Autodesk Inventor part; units mm, degrees
ref_plane "YZ Plane" through (0, 0, 0) normal (1, 0, 0) x (0, 1, 0)
ref_plane "XZ Plane" through (0, 0, 0) normal (0, 1, 0) x (-1, 0, 0)
ref_plane "XY Plane" through (0, 0, 0) normal (0, 0, 1) x (1, 0, 0)
sketch "Sketch1" plane through (0, 0, 0) normal (0, 0, 1) x (1, 0, 0)
  line L0 (3.7674, 2.461) -> (4.3315, 3.068) construction
  line L1 (4.3315, 3.068) -> (2.5, 4.7697) construction
  line L2 (2.5, 4.7697) -> (2.94, 6) construction
  line L3 (2.94, 6) -> (-2, 6) construction
  line L4 (-2, 6) -> (-2, 4.0311) construction
  arc A0 (-2, 4.0311) -> (-3.182, 3.182) centre (0, 0) ccw construction
  line L5 (-3.182, 3.182) -> (-3.182, -3.182) construction
  line L6 (-3.182, -3.182) -> (3.182, -3.182) construction
  arc A1 (3.182, -3.182) -> (3.7674, 2.461) centre (0, 0) ccw construction
  circle A2 centre (0, 0) radius 1.2484
  circle A3 centre (0, 3) radius 0.7934
  circle A4 centre (1.875, -1.75) radius 0.7934
  circle A5 centre (-1.875, -1.75) radius 0.7934
  circle A6 centre (0, 0) radius 4 construction
  line L7 (-2, -4.0311) -> (-2, -3.182) construction
  arc A7 (-2, -4.0311) -> (3.182, -3.182) centre (0, 0) ccw construction
  line L8 (-2, -3.182) -> (3.182, -3.182) construction
  arc A8 (-2, 4.0311) -> (-2, -4.0311) centre (0, 0) ccw construction
  line L9 (-3.182, 3.182) -> (-4.182, 3.182) construction
  line L10 (-4.182, 3.182) -> (-4.182, 4.182) construction
  line L11 (-4.182, 4.182) -> (-3.182, 4.182) construction
  line L12 (-3.182, 4.182) -> (-3.182, 3.182) construction
  line L13 (3.182, -3.182) -> (4.182, -3.182) construction
  line L14 (4.182, -3.182) -> (4.182, -4.182) construction
  line L15 (4.182, -4.182) -> (3.182, -4.182) construction
  line L16 (3.182, -4.182) -> (3.182, -3.182) construction
  line L17 (4.182, -4.182) -> (-4.182, -4.182) construction
  line L18 (-4.182, -4.182) -> (-4.182, -3.182) construction
  line L19 (-4.182, -3.182) -> (4.182, -3.182) construction
  line L20 (4.182, -3.182) -> (4.182, -4.182) construction
  line L21 (-4.182, 4.182) -> (-3.182, 4.182) construction
  line L22 (-3.182, 4.182) -> (-3.182, -4.182) construction
  line L23 (-3.182, -4.182) -> (-4.182, -4.182) construction
  line L24 (-4.182, -4.182) -> (-4.182, 4.182) construction
  line L25 (4.3315, 3.068) -> (6.7138, 5.632) construction
  line L26 (4.3315, 3.068) -> (4.6718, 3.4343) construction
  line L27 (4.6718, 3.4343) -> (2.6832, 5.282) construction
  line L28 (6.7138, 5.632) -> (4.8824, 7.3337) construction
  line L29 (2.5, 4.7697) -> (4.8824, 7.3337) construction
  line L30 (2.8403, 5.136) -> (-3.182, 4.182) construction
  line L31 (4.6718, 3.4343) -> (4.182, -3.182) construction
  circle A9 centre (-3.182, -3.182) radius 0.5 construction
  line L32 (-4.182, 4.182) -> (-4.182, -4.182)
  line L33 (-4.182, -4.182) -> (4.182, -4.182)
  line L34 (4.182, -4.182) -> (4.6718, 3.4343)
  line L35 (6.7138, 5.632) -> (4.6718, 3.4343)
  line L36 (6.7138, 5.632) -> (4.9203, 7.2985)
  line L37 (4.9203, 7.2985) -> (2.8403, 5.136)
  line L38 (2.8403, 5.136) -> (-4.182, 4.182)
  dimension "d0" = 1
  dimension "d1" = 1
  dimension "d2" = 1
  dimension "d3" = 1
  dimension "d4" = 3.5
  dimension "d5" = 0.5
extrude "Extrusion1" add sketch "Sketch1" along normal blind 1
sketch "Sketch2" plane through (0, 0, 1) normal (0, 0, 1) x (1, 0, 0)
  circle A0 centre (0, 0) radius 1.2484
  circle A1 centre (0, 3) radius 0.7934
  line L0 (-3.182, -3.182) -> (3.182, -3.182) construction
  circle A2 centre (0, 0) radius 4 construction
  line L1 (-3.182, 3.182) -> (-3.182, -3.182) construction
  arc A3 (-2, 4.0311) -> (-2, -4.0311) centre (0, 0) ccw construction
  arc A4 (-2, 4.0311) -> (-3.182, 3.182) centre (0, 0) ccw construction
  arc A5 (3.182, -3.182) -> (3.7674, 2.461) centre (0, 0) ccw construction
  line L2 (3.7674, 2.461) -> (4.3315, 3.068) construction
  line L3 (4.3315, 3.068) -> (2.5, 4.7697) construction
  line L4 (-2, -3.182) -> (3.182, -3.182) construction
  arc A6 (-2, -4.0311) -> (3.182, -3.182) centre (0, 0) ccw construction
  line L5 (-2, -4.0311) -> (-2, -3.182) construction
  circle A7 centre (-1.875, -1.75) radius 0.7934
  line L6 (-2, 6) -> (-2, 4.0311) construction
  line L7 (2.5, 4.7697) -> (2.94, 6) construction
  line L8 (2.94, 6) -> (-2, 6) construction
  circle A8 centre (1.875, -1.75) radius 0.7934
  line L9 (-3.182, 3.182) -> (-4.182, 3.182) construction
  line L10 (-4.182, 3.182) -> (-4.182, 4.182) construction
  line L11 (-4.182, 4.182) -> (-3.182, 4.182) construction
  line L12 (-3.182, 4.182) -> (-3.182, 3.182) construction
  line L13 (3.182, -3.182) -> (4.182, -3.182) construction
  line L14 (4.182, -3.182) -> (4.182, -4.182) construction
  line L15 (4.182, -4.182) -> (3.182, -4.182) construction
  line L16 (3.182, -4.182) -> (3.182, -3.182) construction
  line L17 (4.182, -4.182) -> (-4.182, -4.182) construction
  line L18 (-4.182, -4.182) -> (-4.182, -3.182) construction
  line L19 (-4.182, -3.182) -> (4.182, -3.182) construction
  line L20 (4.182, -3.182) -> (4.182, -4.182) construction
  line L21 (-4.182, 4.182) -> (-3.182, 4.182) construction
  line L22 (-3.182, 4.182) -> (-3.182, -4.182) construction
  line L23 (-3.182, -4.182) -> (-4.182, -4.182) construction
  line L24 (-4.182, -4.182) -> (-4.182, 4.182) construction
  line L25 (4.3315, 3.068) -> (6.7138, 5.632) construction
  line L26 (4.3315, 3.068) -> (4.6718, 3.4343) construction
  line L27 (4.6718, 3.4343) -> (2.6832, 5.282) construction
  line L28 (6.7138, 5.632) -> (4.8824, 7.3337) construction
  line L29 (2.5, 4.7697) -> (4.8824, 7.3337) construction
  line L30 (2.8403, 5.136) -> (-3.182, 4.182) construction
  line L31 (4.6718, 3.4343) -> (4.182, -3.182) construction
  arc A9 (-3.182, -2.682) -> (-2.682, -3.182) centre (-3.182, -3.182) ccw
  line L32 (-4.182, 4.182) -> (-4.182, -4.182)
  line L33 (-4.182, -4.182) -> (4.182, -4.182)
  line L34 (4.182, -4.182) -> (4.6718, 3.4343)
  line L35 (6.7138, 5.632) -> (4.6718, 3.4343)
  line L36 (6.7138, 5.632) -> (4.9203, 7.2985)
  line L37 (4.9203, 7.2985) -> (2.8403, 5.136)
  line L38 (2.8403, 5.136) -> (-4.182, 4.182)
  line L39 (-3.182, -2.682) -> (-3.182, 4.3178)
  line L40 (2.8403, 5.136) -> (-4.182, 4.182)
  line L41 (-2.682, -3.182) -> (4.2463, -3.182)
  dimension "d8" = 1
  dimension "d9" = 1
  dimension "d10" = 1
  dimension "d11" = 1
  dimension "d12" = 3.5
  dimension "d13" = 0.5
extrude "Extrusion2" add sketch "Sketch2" along normal blind 2.5 contours A9 L41 L34 L33 L32 L38 L39
sketch "Sketch3" plane through (0, 0, 1) normal (0, 0, 1) x (1, 0, 0)
  circle A0 centre (0, 0) radius 1.2484
  circle A1 centre (0, 3) radius 0.7934
  line L0 (-3.182, -3.182) -> (3.182, -3.182) construction
  circle A2 centre (0, 0) radius 4 construction
  line L1 (-3.182, 3.182) -> (-3.182, -3.182) construction
  arc A3 (-2, 4.0311) -> (-2, -4.0311) centre (0, 0) ccw construction
  arc A4 (-2, 4.0311) -> (-3.182, 3.182) centre (0, 0) ccw construction
  arc A5 (3.182, -3.182) -> (3.7674, 2.461) centre (0, 0) ccw construction
  line L2 (3.7674, 2.461) -> (4.3315, 3.068) construction
  line L3 (4.3315, 3.068) -> (2.5, 4.7697) construction
  line L4 (-2, -3.182) -> (3.182, -3.182) construction
  arc A6 (-2, -4.0311) -> (3.182, -3.182) centre (0, 0) ccw construction
  line L5 (-2, -4.0311) -> (-2, -3.182) construction
  circle A7 centre (-1.875, -1.75) radius 0.7934
  line L6 (-2, 6) -> (-2, 4.0311) construction
  line L7 (2.5, 4.7697) -> (2.94, 6) construction
  line L8 (2.94, 6) -> (-2, 6) construction
  circle A8 centre (1.875, -1.75) radius 0.7934
  line L9 (-3.182, 3.182) -> (-4.182, 3.182) construction
  line L10 (-4.182, 3.182) -> (-4.182, 4.182) construction
  line L11 (-4.182, 4.182) -> (-3.182, 4.182) construction
  line L12 (-3.182, 4.182) -> (-3.182, 3.182) construction
  line L13 (3.182, -3.182) -> (4.182, -3.182) construction
  line L14 (4.182, -3.182) -> (4.182, -4.182) construction
  line L15 (4.182, -4.182) -> (3.182, -4.182) construction
  line L16 (3.182, -4.182) -> (3.182, -3.182) construction
  line L17 (4.182, -4.182) -> (-4.182, -4.182) construction
  line L18 (-4.182, -4.182) -> (-4.182, -3.182) construction
  line L19 (-4.182, -3.182) -> (4.182, -3.182) construction
  line L20 (4.182, -3.182) -> (4.182, -4.182) construction
  line L21 (-4.182, 4.182) -> (-3.182, 4.182) construction
  line L22 (-3.182, 4.182) -> (-3.182, -4.182) construction
  line L23 (-3.182, -4.182) -> (-4.182, -4.182) construction
  line L24 (-4.182, -4.182) -> (-4.182, 4.182) construction
  line L25 (4.3315, 3.068) -> (6.7138, 5.632) construction
  line L26 (4.3315, 3.068) -> (4.6718, 3.4343) construction
  line L27 (4.6718, 3.4343) -> (2.6832, 5.282) construction
  line L28 (6.7138, 5.632) -> (4.8824, 7.3337) construction
  line L29 (2.5, 4.7697) -> (4.8824, 7.3337) construction
  line L30 (2.8403, 5.136) -> (-3.182, 4.182) construction
  line L31 (4.6718, 3.4343) -> (4.182, -3.182) construction
  circle A9 centre (-3.182, -3.182) radius 0.5 construction
  line L32 (-4.182, 4.182) -> (-4.182, -4.182)
  line L33 (-4.182, -4.182) -> (4.182, -4.182)
  line L34 (4.182, -4.182) -> (4.6718, 3.4343)
  line L35 (6.7138, 5.632) -> (4.6718, 3.4343)
  line L36 (6.7138, 5.632) -> (4.9203, 7.2985)
  line L37 (4.9203, 7.2985) -> (2.8403, 5.136)
  line L38 (2.8403, 5.136) -> (-4.182, 4.182)
  line L39 (2.8403, 5.136) -> (-3.182, 4.3178)
  line L40 (4.2463, -3.182) -> (4.6718, 3.4343)
  line L41 (2.8403, 5.136) -> (4.6718, 3.4343)
  dimension "d16" = 1
  dimension "d17" = 1
  dimension "d18" = 1
  dimension "d19" = 1
  dimension "d20" = 3.5
  dimension "d21" = 0.5
extrude "Extrusion3" add sketch "Sketch3" along normal blind 2 contours L37 L36 L35 L41
sketch "Sketch4" plane through (4.9203, 7.2985, 3) normal (0.6807, 0.7326, 0) x (0.7326, -0.6807, 0)
  line L0 (2.4482, 2) -> (-0.0518, 2) construction
  line L1 (2.4482, 2) -> (2.4482, 0) construction
  line L2 (-0.0518, 0) -> (2.4482, 0) construction
  line L3 (-0.0518, 2) -> (-0.0518, 0) construction
  line L4 (2.4482, 0) -> (0, 0) construction
  line L5 (1.2241, 0) -> (-0.0518, 0) construction
  line L6 (-0.0518, 0) -> (-0.0518, 1) construction
  line L7 (-0.0518, 1) -> (1.2241, 1) construction
  line L8 (1.2241, 1) -> (1.2241, 0) construction
  circle A0 centre (1.2241, 1) radius 0.65
  dimension "d24" = 1.3
extrude "Extrusion4" cut sketch "Sketch4" against normal blind 3
sketch "Sketch5" plane through (0, 0, 0) normal (0, 0, -1) x (-1, 0, 0)
  line L0 (4.182, 4.182) -> (4.182, -4.182)
  line L1 (4.182, -4.182) -> (-4.182, -4.182)
  line L2 (-4.182, -4.182) -> (-4.2463, -3.182)
  line L3 (-4.2463, -3.182) -> (2.682, -3.182)
  arc A0 (2.682, -3.182) -> (3.182, -2.682) centre (3.182, -3.182) ccw
  line L4 (3.182, -2.682) -> (3.182, 4.3178)
  line L5 (3.182, 4.3178) -> (4.182, 4.182)
  point P0 (0, 0)
extrude "Extrusion5" add sketch "Sketch5" along normal blind 2.5
sketch "Sketch6" plane through (0, 0, 0) normal (0, 0, -1) x (-1, 0, 0)
  line L0 (-6.7138, 5.632) -> (-4.9203, 7.2985)
  line L1 (-4.9203, 7.2985) -> (-2.8403, 5.136)
  line L2 (-2.8403, 5.136) -> (-4.6718, 3.4343)
  line L3 (-4.6718, 3.4343) -> (-6.7138, 5.632)
  point P0 (0, 0)
extrude "Extrusion6" add sketch "Sketch6" along normal blind 2
sketch "Sketch7" plane through (4.9203, 7.2985, 3) normal (0.6807, 0.7326, 0) x (0.7326, -0.6807, 0)
  line L0 (2.4482, 5) -> (-0.0518, 5)
  circle A0 centre (1.2241, 4) radius 0.65
  point P0 (1.3634, 3)
extrude "Extrusion7" cut sketch "Sketch7" against normal blind 4
sketch "Sketch8" plane through (0, 0, 3.5) normal (0, 0, 1) x (1, 0, 0)
  line L0 (-4.9294, -4.4454) -> (7.7152, -4.4454)
  line L1 (7.7152, -4.4454) -> (7.7152, 7.9918)
  line L2 (7.7152, 7.9918) -> (-4.9294, 7.9918)
  line L3 (-4.9294, 7.9918) -> (-4.9294, -4.4454)
  point P0 (0, 0)
extrude "Extrusion8" cut sketch "Sketch8" against normal blind 2.5
properties part number "MS_Holderv11"
Geometry check sheet. Reference: the model listing, model coordinates, mm. A direction names the side the tool comes from. Round coordinates to 2 decimals unless told otherwise and drop trailing zeros. Write each loop counter-clockwise with the first axis right and the second up, starting at its lowest first coordinate (ties: lowest second). Pieces come first, ordered by that corner, then holes. Notation, with made-up numbers: (7.5, -34.5) - (31.5, -34.5) arc R25 cw to (31.5, -21.5) - close; hole circle Ø5 at (27, -34). An arc over 180 degrees is marked (long way). One line per item, written item: value.
1. Cross-section at B-B on z = 0.75. Give the number of separate pieces and of enclosed holes in the cut face, and give its area (3 significant figures).
The answers:
separate pieces: 1
enclosed holes: 4
area: 72.3 mm^2
2. Set-up check for faces 5 (the face through (1, -3.182, -1)), 6 (the face through (-3.55, -3.52, -1.23)), 7 (the face through (0, 2, 1)): record each of +Z, -Z, +X, -X, +Y, -Y from which the full face is reachable in a straight line by a thin tool's end or side.
The answers:
face 5: -Z, +X
face 6: -Z
face 7: +Z, +X, -X, +Y, -Y
3. Scan lines: L1, parallel to X at y = -1.5, z = 0.75; L2, parallel to Y at x = 0, z = 0.7; L3, parallel to X at y = -2, z = 0.1. Record each from-to range of solid material in increasing order.
The answers:
L1: x = -4.18 to -2.63, -1.12 to 1.12, 2.63 to 4.35
L2: y = -4.18 to -1.25, 1.25 to 2.21, 3.79 to 4.75
L3: x = -4.18 to -2.63, -1.12 to 1.12, 2.63 to 4.32
4. Mould release check, pull along Y, two halves, no side actions. Record for faces 1 (the face through (-1.5, -3.4, -2.5)), 2 (the face through (5.83, 6.454, -0.146)), 3 (the face through (5.066, 5.144, -1.548)), 4 (the face through (1, 1, 0)): released by +Y, released by -Y, zero draft, split by the parting line, or undercut.
The answers:
face 1: zero draft
face 2: released by +Y
face 3: undercut
face 4: undercut
5. Cross-section at C-C on x = 0. Record the boundary of the cut face in (y, z), and give its area (3 significant figures).
The answers:
outline: (-4.18, -2.5) - (-3.18, -2.5) - (-3.18, 0) - (-1.25, 0) - (-1.25, 1) - (-4.18, 1) - close; (1.25, 0) - (2.21, 0) - (2.21, 1) - (1.25, 1) - close; (3.79, 0) - (4.75, 0) - (4.75, 1) - (3.79, 1) - close
area: 7.35 mm^2
6. Depth check by flat-ended pin: pin 1 Ø3 at (x, y) = (5, 4.5) entering from -Z; pin 2 Ø2.5 at (x, y) = (1, 2.5) entering from -Z; pin 3 Ø1.2 at (x, z) = (2, -1) entering from +Y. Enter the tip coordinate at first touch or a pass-through.
The answers:
pin 1: stops at z = -2
pin 2: stops at z = 0
pin 3: stops at y = -3.18
7. Cross-section at D-D on y = 0. Record the boundary of the cut face in (x, z).
The answers:
outline: (-4.18, -2.5) - (-3.18, -2.5) - (-3.18, 0) - (-1.25, 0) - (-1.25, 1) - (-4.18, 1) - close; (1.25, 0) - (4.45, 0) - (4.45, 1) - (1.25, 1) - close
8. Cross-section at A-A on z = -1.85. Record the boundary of the cut face in (x, y), and give its area (3 significant figures).
The answers:
outline: (-4.18, -4.18) - (4.18, -4.18) - (4.25, -3.18) - (-2.68, -3.18) arc R0.5 cw (long way) to (-3.18, -2.68) - (-3.18, 4.32) - (-4.18, 4.18) - close; (2.84, 5.14) - (4.67, 3.43) - (6.71, 5.63) - (4.92, 7.3) - close
area: 22.7 mm^2
